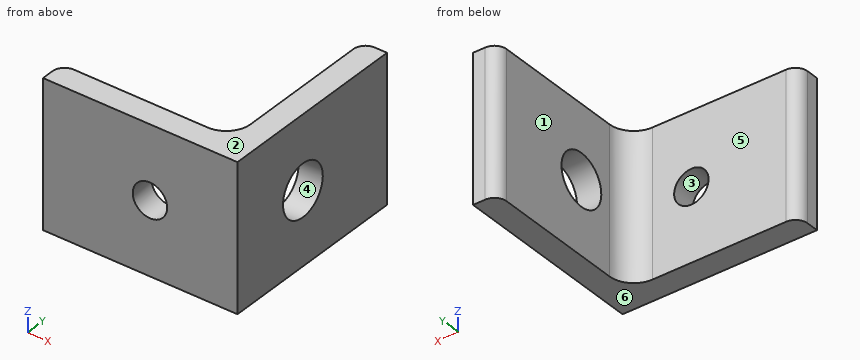
```python
from build123d import *

# Parameters (mm, degrees)
BOSS_EXTRUDE1_DEPTH     = 9.525
F_1_4_CLEARANCE_HOLE1_D = 6.7564
F_8_CLEARANCE_HOLE1_D   = 4.4958


with BuildPart() as part:
    # Sketch2 → Boss-Extrude1 (new, symmetric)
    with BuildSketch(Plane.XY):
        with BuildLine():
            Line((-12.7, 0), (12.7, 0))
            Line((12.7, 0), (12.7, 25.4))
            Line((12.7, 25.4), (11.1125, 25.4))
            ThreePointArc((11.1125, 25.4), (9.989967985, 24.935032015), (9.525, 23.8125))
            Line((9.525, 23.8125), (9.525, 6.35))
            ThreePointArc((9.525, 6.35), (8.59506403, 4.10493597), (6.35, 3.175))
            Line((6.35, 3.175), (-11.1125, 3.175))
            ThreePointArc((-11.1125, 3.175), (-12.235032015, 2.710032015), (-12.7, 1.5875))
            Line((-12.7, 1.5875), (-12.7, 0))
        make_face()
    extrude(amount=BOSS_EXTRUDE1_DEPTH, both=True)

    # 1/4 Clearance Hole1 (through all)
    with Locations(Plane.ZY.offset(-9.525)):
        with Locations((0, 11.1166148)):
            Hole(F_1_4_CLEARANCE_HOLE1_D / 2)

    # #8 Clearance Hole1 (through all)
    with Locations(Plane(origin=(0, 3.175, 0), x_dir=(1, 0, 0), z_dir=(0, 1, 0))):
        with Locations((1.27, 0)):
            Hole(F_8_CLEARANCE_HOLE1_D / 2)


solid = part.part
```
Could you check a few things on this model? Use its own coordinates, in mm. Face numbers are marked on the shaded views. A direction names the side the tool comes from. Round coordinates to 2 decimals unless told otherwise and drop trailing zeros. Loops run counter-clockwise (first coordinate to the right, second up) from the corner with the lowest first, then second, coordinate; pieces in that order, holes last. Notation, with made-up numbers: M 45.5,25.5 L 90.5,25.5 A27 ccw 90.5,44.5 Z; hole C 32,47 d9. An arc over 180 degrees is marked long. Answer as CSV lines item,"result".
1) For pin 1 Ø8.5 at (y, z) = (18.5, -0.5) entering from -X (3 decimals); pin 2 Ø6 at (x, z) = (5.5, 3.5) entering from +Y; pin 3 Ø6 at (y, z) = (11.12, 0) entering from +X, each with a flat end and sliding along its axis, tell me the tip position at first contact or that it passes through.
From the geometry:
pin 1,"x = 9.525"
pin 2,"y = 4.01"
pin 3,"through"
2) Imagine slicing it at A-A on x = 1.27. List the corners of the cut face in (y, z) for me (3 decimals).
From the geometry:
outline,"M 0,-9.525 L 3.175,-9.525 L 3.175,-2.248 L 0,-2.248 Z; M 0,2.248 L 3.175,2.248 L 3.175,9.525 L 0,9.525 Z"
3) We'd pull the mould along Z, two halves only. Please class the marked faces 3, 4, 5 and 6: released by +Z, released by -Z, zero draft, split by the parting line, or undercut.
From the geometry:
face 3,"undercut"
face 4,"undercut"
face 5,"zero draft"
face 6,"released by -Z"
4) Imagine slicing it at D-D on x = -4.5. List the corners of the cut face in (y, z) for me (3 decimals).
From the geometry:
outline,"M 0,-9.525 L 3.175,-9.525 L 3.175,9.525 L 0,9.525 Z"
5) If I drill on probe 1 along Y at (x, z) = (11, 0); probe 2 along Z at (x, y) = (1.27, 1.95) (3 decimals); probe 3 along Y at (x, z) = (-1, -2) (3 decimals), over which ranges is the centre line in solid material (lowest first)?
From the geometry:
probe 1,"0 to 7.74, 14.49 to 25.4"
probe 2,"-9.525 to -2.248, 2.248 to 9.525"
probe 3,"0 to 3.175"
6) Imagine slicing it at C-C on x = 10.75. List the corners of the cut face in (y, z) for me (3 decimals), and give its area (3 significant figures).
From the geometry:
outline,"M 0,-9.525 L 25.358,-9.525 L 25.358,9.525 L 0,9.525 Z; hole C 11.117,0 d6.756"
area,"447 mm^2"
7) Which directions (+Z, -Z, +X, -X, +Y, -Y) give clear straight access to the entire face, cutting with the end or side of a thin tool? Please do the marked faces 1 and 2.
From the geometry:
face 1,"+Z, -Z, -X, +Y"
face 2,"+Z, +X, -X, +Y, -Y"
